Geometry check sheet. Reference: the model listing, model coordinates, mm. A direction names the side the tool comes from. Give positions to 0.01 mm unless a question says otherwise; leave off trailing zeros. Write each loop counter-clockwise with the first axis right and the second up, starting at its lowest first coordinate (ties: lowest second). Pieces come first, ordered by that corner, then holes. Notation, with made-up numbers: (60.5, -28) -> (65.5, -28) arc R17 cw to (65.5, -14) -> close; hole circle Ø8 at (10, -26.75). An arc over 180 degrees is marked (long way). One line per item, written item: value.
from build123d import *

# Parameters (mm, degrees)
SKETCH1_R               = 55
BOSS_EXTRUDE1_DEPTH     = 7.5
SKETCH2_R               = 20
BOSS_EXTRUDE2_DEPTH     = 273
SKETCH3_R               = 14
BOSS_EXTRUDE3_DEPTH     = 22
SKETCH4_R               = 53
CUT_EXTRUDE1_DEPTH      = 3
SKETCH5_R               = 6
CUT_EXTRUDE2_DEPTH      = 317.700173666
CUT_EXTRUDE3_DEPTH      = 313.339959019
CUT_EXTRUDE3_DEPTH_BACK = 313.339959019
SKETCH7_R               = 3
M3_TAPPED_HOLE1_D       = 2.5
M3_TAPPED_HOLE1_DEPTH   = 8
M3_TAPPED_HOLE1_TIP     = 0.751075774


with BuildPart() as part:
    # Sketch1 → Boss-Extrude1 (new, symmetric)
    with BuildSketch(Plane(origin=(0, 0, 0), x_dir=(1, 0, 0), z_dir=(0, 1, 0))):
        with Locations(Location((0, 0, 0), (0, 0, 270))):
            Circle(SKETCH1_R)
    extrude(amount=BOSS_EXTRUDE1_DEPTH, both=True)

    # Sketch2 → Boss-Extrude2 (add)
    with BuildSketch(Plane(origin=(0, 7.5, 0), x_dir=(1, 0, 0), z_dir=(0, 1, 0))):
        with Locations(Location((0, 0, 0), (0, 0, 270))):
            Circle(SKETCH2_R)
    extrude(amount=BOSS_EXTRUDE2_DEPTH)

    # Sketch3 → Boss-Extrude3 (add)
    with BuildSketch(Plane(origin=(0, 280.5, 0), x_dir=(1, 0, 0), z_dir=(0, 1, 0))):
        with Locations(Location((0, 0, 0), (0, 0, 270))):
            Circle(SKETCH3_R)
    extrude(amount=BOSS_EXTRUDE3_DEPTH)

    # Sketch4 → Cut-Extrude1 (cut)
    with BuildSketch(Plane.XZ.offset(7.5)):
        with Locations(Location((0, 0, 0), (0, 0, 270))):
            Circle(SKETCH4_R)
    extrude(amount=-CUT_EXTRUDE1_DEPTH, mode=Mode.SUBTRACT)

    # Sketch5 → Cut-Extrude2 (cut, through all)
    with BuildSketch(Plane.XZ.offset(4.5)):
        with Locations(Location((0, 0, 0), (0, 0, 270))):
            Circle(SKETCH5_R)
    extrude(amount=-CUT_EXTRUDE2_DEPTH, mode=Mode.SUBTRACT)

    # Sketch7 → Cut-Extrude3 (cut, two sides: drawn at the far end of the back side and taken through both)
    with BuildSketch(Plane.XY.offset(-CUT_EXTRUDE3_DEPTH_BACK)):
        with Locations((0, 291.5)):
            Circle(SKETCH7_R)
    extrude(amount=CUT_EXTRUDE3_DEPTH + CUT_EXTRUDE3_DEPTH_BACK, mode=Mode.SUBTRACT)

    # M3 Tapped Hole1
    with Locations(Plane(origin=(0, 7.5, 0), x_dir=(1, 0, 0), z_dir=(0, 1, 0))):
        with Locations((-20.56810334, -11.875), (20.56810334, -11.875), (0, 23.75)):
            Hole(M3_TAPPED_HOLE1_D / 2, depth=M3_TAPPED_HOLE1_DEPTH)
            with Locations((0, 0, -(M3_TAPPED_HOLE1_DEPTH + M3_TAPPED_HOLE1_TIP / 2))):  # 118° drill point
                Cone(0, M3_TAPPED_HOLE1_D / 2, M3_TAPPED_HOLE1_TIP, mode=Mode.SUBTRACT)


solid = part.part
1) Sectioned sample at D-D on z = -40. Record the cut outline in (x, y).
Verdict:
outline: (-37.75, -7.5) -> (-34.77, -7.5) -> (-34.77, -4.5) -> (34.77, -4.5) -> (34.77, -7.5) -> (37.75, -7.5) -> (37.75, 7.5) -> (-37.75, 7.5) -> close
2) Depth check by flat-ended pin: pin 1 Ø8 at (x, z) = (-13, -31.5) entering from -Y; pin 2 Ø4 at (x, z) = (-20.57, 11.88) entering from +Y. Enter the tip coordinate at first touch or a pass-through.
Verdict:
pin 1: y = -4.5
pin 2: y = 7.5
3) Tool access check on faces 4 (the flat face through (-24, 7.5, -1)), 5 (the flat face through (1, -4.5, -11)), 6 (the cylindrical face through (1.802, 146.851, -5.723)). Record the directions out of +Z, -Z, +X, -X, +Y, -Y that give a thin tool (end or side, any length) a straight path to the whole face; none if there is none.
Verdict:
face 4: +Y
face 5: -Y
face 6: +Y, -Y
4) Sectioned sample at A-A on z = 0. Record the cut outline in (x, y), plus the area to 3 significant figures.
Verdict:
outline: (-55, -7.5) -> (-53, -7.5) -> (-53, -4.5) -> (-6, -4.5) -> (-6, 302.5) -> (-14, 302.5) -> (-14, 280.5) -> (-20, 280.5) -> (-20, 7.5) -> (-55, 7.5) -> close; (6, -4.5) -> (53, -4.5) -> (53, -7.5) -> (55, -7.5) -> (55, 7.5) -> (20, 7.5) -> (20, 280.5) -> (14, 280.5) -> (14, 302.5) -> (6, 302.5) -> close
area: 9,180 mm^2
5) Scan lines: probe 1 along Y at (x, z) = (0, -8.5); probe 2 along X at (y, z) = (291.5, 11.5); probe 3 along X at (y, z) = (291.5, 12). Record each from-to range of solid material in increasing order.
Verdict:
probe 1: -4.5 to 288.5, 294.5 to 302.5
probe 2: -7.98 to -3, 3 to 7.98
probe 3: -7.21 to -3, 3 to 7.21
6) Mould release check, pull along X, two halves, no side actions. Record for faces 1 (the cylindrical face through (-3, 291.6, -9.7)), 2 (the flat face through (14, 280.5, 4)), 3 (the cylindrical face through (-5.362, 291.346, 12.932)): released by +X, released by -X, zero draft, split by the parting line, or undercut.
Verdict:
face 1: undercut
face 2: zero draft
face 3: split by the parting line
7) Sectioned sample at B-B on y = 291.5. Record the cut outline in (x, z).
Verdict:
outline: (-3, -13.67) -> (-3, -5.2) arc R6 cw to (-3, 5.2) -> (-3, 13.67) arc R14 ccw to start; (3, -13.67) arc R14 ccw to (3, 13.67) -> (3, 5.2) arc R6 cw to (3, -5.2) -> close
8) Sectioned sample at C-C on x = 28.5. Record the cut outline in (y, z) (3 decimals), plus the area to 3 significant figures.
Verdict:
outline: (-7.5, -47.04) -> (7.5, -47.04) -> (7.5, 47.04) -> (-7.5, 47.04) -> (-7.5, 44.685) -> (-4.5, 44.685) -> (-4.5, -44.685) -> (-7.5, -44.685) -> close
area: 1,140 mm^2
